Verification items for the finished model (mm, model axes). Round coordinates to 2 decimals unless told otherwise and drop trailing zeros. Write each loop counter-clockwise with the first axis right and the second up, starting at its lowest first coordinate (ties: lowest second). Pieces come first, ordered by that corner, then holes. Notation, with made-up numbers: M -13.5,7 L 19.5,7 A24 ccw 19.5,21 Z; hole C 36,10.5 d6. An arc over 180 degrees is marked long. One line per question, with ' | ' between items.
from build123d import *

# Parameters (mm, degrees)
F1_DEPTH = 2.5
F2_D     = 3.3
F2_DEPTH = 40
F2_TIP   = 0.9914200214


with BuildPart() as f1:
    # F0 (on Front) → F1 (new body)
    with BuildSketch(Plane.XZ):
        Polygon((0, -400), (0, 0), (330, 0), (330, -400), (350, -400), (350, 200), (-20, 200), (-20, -400), align=None)
    extrude(amount=F1_DEPTH)

    # F2
    with Locations(Plane(origin=(0, 0, 0), x_dir=(1, 0, 0), z_dir=(0, 1, 0))):
        with Locations((-9, 100), (-9, 200), (-9, 300), (-9, 125), (-9, 225), (-9, 325)):
            Hole(F2_D / 2, depth=F2_DEPTH)
            with Locations((0, 0, -(F2_DEPTH + F2_TIP / 2))):  # 118° drill point
                Cone(0, F2_D / 2, F2_TIP, mode=Mode.SUBTRACT)


solid = f1.part
1. Section check A-A, the plane z = -84. Record the cut outline in (x, y), then the cut area to 3 significant figures.
Results:
outline: M -20,-2.5 L 0,-2.5 L 0,0 L -20,0 Z; M 330,-2.5 L 350,-2.5 L 350,0 L 330,0 Z | area: 100 mm2
2. Thickness scan on line 1 (X direction, y = -1.3, z = -325); line 2 (X direction, y = -1.9, z = -331.5); line 3 (Z direction, x = 307.5, y = -1.8). Record the ranges inside material, lowest first.
Results:
line 1: x = -20 to -10.65, -7.35 to 0, 330 to 350 | line 2: x = -20 to 0, 330 to 350 | line 3: z = 0 to 200
3. Go/stop test with flat-tipped pins: P1, Ø0.8, axis at x = 199.5, y = -1, coming from the -Z side; P2, Ø4, axis at x = -9, z = -100, coming from the -Y side. Record where each tip stops, or that it passes through.
Results:
P1: stops at z = 0 | P2: stops at y = -2.5
4. Section check C-C, the plane x = 252.5. Record the cut outline in (y, z), then the cut area to 3 significant figures.
Results:
outline: M -2.5,0 L 0,0 L 0,200 L -2.5,200 Z | area: 500 mm2
5. Section check B-B, the plane y = -2.05. Record the cut outline in (x, z).
Results:
outline: M -20,-400 L 0,-400 L 0,0 L 330,0 L 330,-400 L 350,-400 L 350,200 L -20,200 Z; hole C -9,-325 d3.3; hole C -9,-300 d3.3; hole C -9,-225 d3.3; hole C -9,-200 d3.3; hole C -9,-125 d3.3; hole C -9,-100 d3.3
